from build123d import *

# Parameters (mm, degrees)
SKIZZE1_R                       = 8.5
AUFSATZ_LINEAR_AUSTRAGEN1_DEPTH = 1.5
SKIZZE2_R                       = 5.9
AUFSATZ_LINEAR_AUSTRAGEN2_DEPTH = 7
SKIZZE3_R                       = 5.9
AUFSATZ_LINEAR_AUSTRAGEN3_DEPTH = 7
SCHNITT_LINEAR_AUSTRAGEN1_DEPTH = 21.820662814
FASE1_SIZE                      = 0.5


with BuildPart() as part:
    # Skizze1 → Aufsatz-Linear austragen1 (new, symmetric)
    with BuildSketch(Plane(origin=(0, 0, 0), x_dir=(1, 0, 0), z_dir=(0, 1, 0))):
        with Locations(Location((0, 0, 0), (0, 0, 270))):
            Circle(SKIZZE1_R)
    extrude(amount=AUFSATZ_LINEAR_AUSTRAGEN1_DEPTH, both=True)

    # Skizze2 → Aufsatz-Linear austragen2 (add)
    with BuildSketch(Plane(origin=(0, 1.5, 0), x_dir=(1, 0, 0), z_dir=(0, 1, 0))):
        with Locations(Location((1, 0, 0), (0, 0, 270))):
            Circle(SKIZZE2_R)
    extrude(amount=AUFSATZ_LINEAR_AUSTRAGEN2_DEPTH)

    # Skizze3 → Aufsatz-Linear austragen3 (add)
    with BuildSketch(Plane.XZ.offset(1.5)):
        with Locations(Location((-1, 0, 0), (0, 0, 270))):
            Circle(SKIZZE3_R)
    extrude(amount=AUFSATZ_LINEAR_AUSTRAGEN3_DEPTH)

    # Skizze4 → Schnitt-Linear austragen1 (cut, through all)
    with BuildSketch(Plane(origin=(0, 8.5, 0), x_dir=(1, 0, 0), z_dir=(0, 1, 0))):
        with BuildLine():
            Line((-2.856571371, -2.8), (2.856571371, -2.8))
            ThreePointArc((2.856571371, -2.8), (0, 4), (-2.856571371, -2.8))
        make_face()
    extrude(amount=-SCHNITT_LINEAR_AUSTRAGEN1_DEPTH, mode=Mode.SUBTRACT)

    # Fase1
    fase1_edges = [part.edges().sort_by_distance(p)[0] for p in [
        (0, -8.5, -4),
        (0, -8.5, 2.8),
        (0, 8.5, -4),
        (0, 8.5, 2.8),
    ]]
    chamfer(fase1_edges, length=FASE1_SIZE)


solid = part.part
Source: CAD feature listing. Evaluate the final solid. Frame: model axes, mm. A direction names the side the tool comes from. Round coordinates to 2 decimals unless told otherwise and drop trailing zeros. Order: outer loops, then holes, each group sorted by start corner. A loop starts at its lowest first (then second) coordinate and runs counter-clockwise, first axis right, second up. Notation, with made-up numbers: (30, -35.5) - (73, -35.5) arc R25 cw to (73, -10.5) - close; hole circle Ø10 at (-3, 5.25). An arc over 180 degrees is marked (long way). Use a Markdown table: item, result. Add a question column.
1. Section query C-C (y = 1.25). Return the cut outline in (x, z), then the cut area to 3 significant figures.
2. Section query B-B (x = 0). Return the cut outline in (y, z).
3. Section query A-A (z = 0). Return the cut outline in (x, y), then the cut area to 3 significant figures.
4. Set-up query: faces 4 (the flat face through (4, -1.5, 4)), 5 (the cylindrical face through (0, 0, -4)), 6 (the flat face through (-4, 1.5, 4)). Return all of +Z, -Z, +X, -X, +Y, -Y with unobstructed straight access to the full face (end or side cutting, diameter ignored); none if empty.
5. Line query: probe 1 along X at (y, z) = (4, 0); probe 2 along Y at (x, z) = (7, -1.25); probe 3 along X at (y, z) = (0, 0). Output: solid intervals per line, ascending.
6. First-contact query: pin 1 (4 mm diameter, centred on y = 5, z = -3.5, fed in from -X); pin 2 (5 mm diameter, centred on y = 5, z = -4.5, fed in from +X); pin 3 (5 mm diameter, centred on y = 1.5, z = 3.5, fed in from -X). Flat tips, straight axial feed; report the tip coordinate or a pass-through.
7. Mould query, pull axis Z, two halves, no side actions, for faces 1 (the flat face through (0, 0, 2.8)), 2 (the cylindrical face through (-4.59, -4.95, 4.68)), 3 (the flat face through (-5, -8.5, 1)). Classes: +Z half, -Z half, draft (parallel to the pull), parting line (faces both ways), or undercut.
8. Section query D-D (x = -6). Return the cut outline in (y, z), then the cut area to 3 significant figures.
Derived:
| question | item | result |
|---|---|---|
| 1 | outline | circle Ø17 at (0, 0); hole (-2.86, 2.8) arc R4 ccw (long way) to (2.86, 2.8) - close |
| 1 | area | 181 mm2 |
| 2 | outline | (-8.5, -5.81) - (-1.5, -5.81) - (-1.5, -8.5) - (1.5, -8.5) - (1.5, -5.81) - (8.5, -5.81) - (8.5, -4.5) - (8, -4) - (-8, -4) - (-8.5, -4.5) - close; (-8.5, 3.3) - (-8, 2.8) - (8, 2.8) - (8.5, 3.3) - (8.5, 5.81) - (1.5, 5.81) - (1.5, 8.5) - (-1.5, 8.5) - (-1.5, 5.81) - (-8.5, 5.81) - close |
| 3 | outline | (-8.5, -1.5) - (-6.9, -1.5) - (-6.9, -8.5) - (-4.5, -8.5) - (-4, -8) - (-4, 8) - (-4.5, 8.5) - (-4.9, 8.5) - (-4.9, 1.5) - (-8.5, 1.5) - close; (4, -8) - (4.5, -8.5) - (4.9, -8.5) - (4.9, -1.5) - (8.5, -1.5) - (8.5, 1.5) - (6.9, 1.5) - (6.9, 8.5) - (4.5, 8.5) - (4, 8) - close |
| 3 | area | 79.7 mm2 |
| 4 | face 4 | -Y |
| 4 | face 5 | +Y, -Y |
| 4 | face 6 | +Y |
| 5 | probe 1 | -4.9 to -4, 4 to 6.9 |
| 5 | probe 2 | -1.5 to 1.5 |
| 5 | probe 3 | -8.5 to -4, 4 to 8.5 |
| 6 | pin 1 | x = -4.71 |
| 6 | pin 2 | x = 6.55 |
| 6 | pin 3 | x = -8.44 |
| 7 | face 1 | undercut |
| 7 | face 2 | parting line |
| 7 | face 3 | draft |
| 8 | outline | (-8.5, -3.13) - (-1.5, -3.13) - (-1.5, -6.02) - (1.5, -6.02) - (1.5, 6.02) - (-1.5, 6.02) - (-1.5, 3.13) - (-8.5, 3.13) - close |
| 8 | area | 80.0 mm2 |
